```python
from build123d import *

# Parameters (mm, degrees)
BOSS_EXTRUDE4_DEPTH = 6


with BuildPart() as part:
    # Sketch5 → Boss-Extrude4 (new body)
    with BuildSketch(Plane.XY):
        with BuildLine():
            Line((0, 31.5), (14, 31.5))
            Line((14, 31.5), (14, 23.5))
            Line((14, 23.5), (11.5, 20.5))
            Line((11.5, 20.5), (10, 25))
            Line((10, 25), (9, 25))
            Line((9, 25), (9, -10))
            Line((9, -10), (2, -10))
            Line((2, -10), (2, -17.5))
            Line((2, -17.5), (6.55, -18.930908802))
            ThreePointArc((6.55, -18.930908802), (8.498478182, -17.432449005), (6.423076923, -16.115384615))
            Line((6.423076923, -16.115384615), (5.961538462, -16.307692308))
            ThreePointArc((5.961538462, -16.307692308), (2.51090022, -14.2332001), (5.516159308, -11.55386436))
            Line((5.516159308, -11.55386436), (10, -12.5))
            Line((10, -12.5), (10, -9))
            Line((10, -9), (12, -6.5))
            Line((12, -6.5), (14, -8.5))
            Line((14, -8.5), (14, -51.5))
            Line((14, -51.5), (6, -51.5))
            Line((6, -51.5), (6, -48.5))
            Line((6, -48.5), (10, -48.5))
            Line((10, -48.5), (10, -35.5))
            Line((10, -35.5), (6.021836686, -37.28163314))
            ThreePointArc((6.021836686, -37.28163314), (2.518102723, -34.699690318), (6.536534963, -33.027929944))
            Line((6.536534963, -33.027929944), (6.436915421, -32.8903006))
            ThreePointArc((6.436915421, -32.8903006), (8.498796421, -31.560077342), (6.55, -30.069091198))
            Line((6.55, -30.069091198), (2, -31.5))
            Line((2, -31.5), (2, -38.5))
            Line((2, -38.5), (0, -38.5))
            Line((0, -38.5), (0, 31.5))
        make_face()
        with BuildLine():
            Line((10, -13.5), (10, -34.5))
            Line((10, -34.5), (5.613102012, -36.368979884))
            ThreePointArc((5.613102012, -36.368979884), (3.510861634, -34.819814191), (5.921920978, -33.816757966))
            Line((5.921920978, -33.816757966), (6.061525702, -33.817167666))
            ThreePointArc((6.061525702, -33.817167666), (9.498478082, -31.587219699), (6.225393962, -29.123030188))
            Line((6.225393962, -29.123030188), (2, -30.5))
            Line((2, -30.5), (2, -18.5))
            Line((2, -18.5), (6.225393962, -19.876969812))
            ThreePointArc((6.225393962, -19.876969812), (9.498012054, -17.400321638), (6.038461538, -15.192307692))
            Line((6.038461538, -15.192307692), (5.576923077, -15.384615385))
            ThreePointArc((5.576923077, -15.384615385), (3.50685843, -14.143276833), (5.303094113, -12.530941132))
            Line((5.303094113, -12.530941132), (10, -13.5))
        make_face(mode=Mode.SUBTRACT)
    extrude(amount=BOSS_EXTRUDE4_DEPTH)


solid = part.part
```
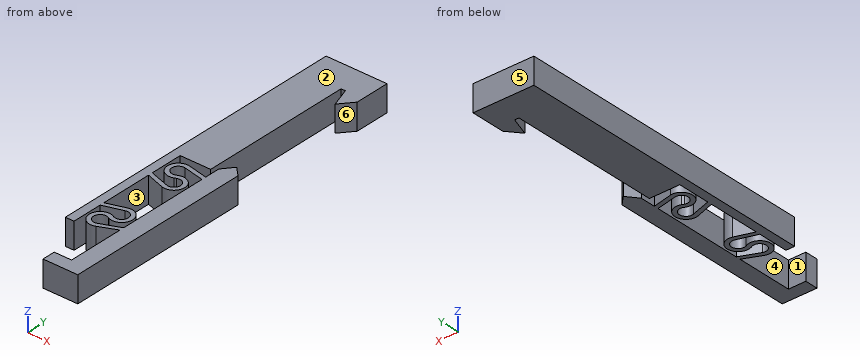
Verification items for the finished model (mm, model axes). Face numbers are marked on the shaded views. A direction names the side the tool comes from. Round coordinates to 2 decimals unless told otherwise and drop trailing zeros. Order: outer loops, then holes, each group sorted by start corner. A loop starts at its lowest first (then second) coordinate and runs counter-clockwise, first axis right, second up. Notation, with made-up numbers: (16.25, 70.5) - (30.25, 70.5) arc R33 cw to (30.25, 102.5) - close; hole circle Ø2 at (28, -9.5). An arc over 180 degrees is marked (long way). Use CSV: the item, a comma, the result in double quotes. Start each with the question number.
1) Thickness scan on L1, parallel to X at y = -14, z = 2.6; L2, parallel to X at y = -28.5, z = 2.65; L3, parallel to X at y = -35, z = 2.1. Record the ranges inside material, lowest first.
2) Access from +Z, -Z, +X, -X, +Y, -Y to the whole of each face (thin tool, end or side, straight path). Record for the marked faces 1, 2 and 3.
3) Go/stop test with flat-tipped pins: P1, Ø3.5, axis at y = -49.5, z = 2.5, coming from the -X side; P2, Ø1, axis at x = 3.5, z = 2.5, coming from the -Y side; P3, Ø2, axis at x = 1, z = 2, coming from the -Y side. Record where each tip stops, or that it passes through.
4) Mould release check, pull along X, two halves, no side actions. Record for the marked faces 4, 5 and 6: +X half, -X half, draft (parallel to the pull), parting line (faces both ways), or undercut.
5) Section check A-A, the plane y = 15. Record the cut outline in (x, z).
Answers:
1,L1,"x = 0 to 2, 2.5 to 3.5, 10 to 14"
1,L2,"x = 0 to 2, 10 to 14"
1,L3,"x = 0 to 2, 2.5 to 3.5, 8.83 to 14"
2,face 1,"+Z, -Z, -X"
2,face 2,"+Z, +X, -X, +Y, -Y"
2,face 3,"+Z, -Z"
3,P1,"stops at x = 6"
3,P2,"stops at y = -37.29"
3,P3,"stops at y = -38.5"
4,face 4,"undercut"
4,face 5,"draft"
4,face 6,"+X half"
5,outline,"(0, 0) - (9, 0) - (9, 6) - (0, 6) - close"
